from build123d import *

# Parameters (mm, degrees)
SKETCH1_W           = 400
SKETCH1_H           = 20
BOSS_EXTRUDE1_DEPTH = 7.5
SKETCH2_R           = 2.5
BOSS_EXTRUDE2_DEPTH = 75
SKETCH3_R           = 2.5
BOSS_EXTRUDE3_DEPTH = 75
SKETCH5_R           = 10
BOSS_EXTRUDE4_DEPTH = 5
BOSS_EXTRUDE5_START = 20
SKETCH6_R           = 10
BOSS_EXTRUDE5_DEPTH = 20
SKETCH7_R           = 8
CUT_EXTRUDE1_DEPTH  = 15


with BuildPart() as part:
    # Sketch1 → Boss-Extrude1 (new body)
    with BuildSketch(Plane(origin=(0, 0, 0), x_dir=(1, 0, 0), z_dir=(0, 1, 0))):
        Rectangle(SKETCH1_W, SKETCH1_H)
        Polygon((200, 10), (0, 20), (-200, 10), align=None)
        Polygon((0, -20), (-200, -10), (200, -10), align=None)
    extrude(amount=BOSS_EXTRUDE1_DEPTH)

    # Sketch2 → Boss-Extrude2 (add)
    with BuildSketch(Plane(origin=(200, 0, 0), x_dir=(0, 0, -1), z_dir=(1, 0, 0))):
        with Locations((0, 3.296264787)):
            Circle(SKETCH2_R)
    extrude(amount=BOSS_EXTRUDE2_DEPTH)

    # Sketch3 → Boss-Extrude3 (add)
    with BuildSketch(Plane.ZY.offset(200)):
        with Locations((0, 3.469116297)):
            Circle(SKETCH3_R)
    extrude(amount=BOSS_EXTRUDE3_DEPTH)

    # Sketch5 → Boss-Extrude4 (add)
    with BuildSketch(Plane(origin=(0, 7.5, 0), x_dir=(1, 0, 0), z_dir=(0, 1, 0))):
        with Locations(Location((0, 0, 0), (0, 0, 270))):
            Circle(SKETCH5_R)
    extrude(amount=BOSS_EXTRUDE4_DEPTH)

    # Sketch6 → Boss-Extrude5 (add)
    with BuildSketch(Plane.XZ.offset(BOSS_EXTRUDE5_START)):
        with Locations(Location((0, 0, 0), (0, 0, 90))):
            Circle(SKETCH6_R)
    extrude(amount=-BOSS_EXTRUDE5_DEPTH)

    # Sketch7 → Cut-Extrude1 (cut)
    with BuildSketch(Plane(origin=(0, -20, 0), x_dir=(-1, 0, 0), z_dir=(0, -1, 0))):
        with Locations(Location((0, 0, 0), (0, 0, 90))):
            Circle(SKETCH7_R)
    extrude(amount=-CUT_EXTRUDE1_DEPTH, mode=Mode.SUBTRACT)


solid = part.part
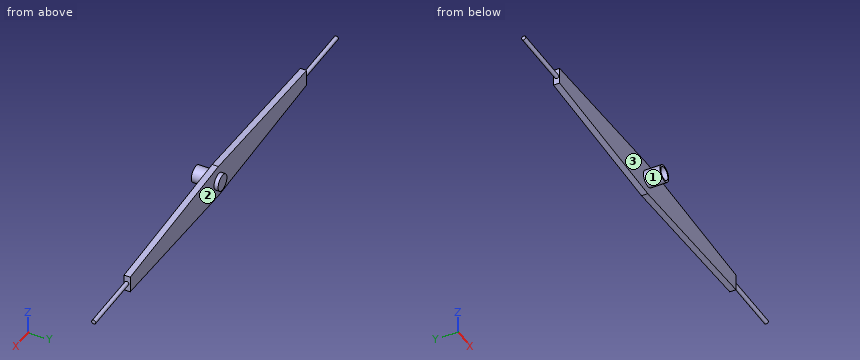
Design review of the part built by this model. Coordinates are the model's own, in mm. Face numbers are marked on the shaded views. Give positions to 0.01 mm unless a question says otherwise; leave off trailing zeros. Write each loop counter-clockwise with the first axis right and the second up, starting at its lowest first coordinate (ties: lowest second). Pieces come first, ordered by that corner, then holes. Notation, with made-up numbers: M 40,62 L 91,62 A6 ccw 91,72 Z; hole C 19.5,22.25 d9. An arc over 180 degrees is marked long. Return JSON: item names as keys, results as strings. Group by question number.
Item 1: Take a section at A-A (x = -34). Give the boundary of the cut face in (y, z).
Item 2: Take a section at B-B (z = 14.5). Give the boundary of the cut face in (x, y).
Item 3: Wall thickness on line 1 along X through (y, z) = (-11.5, 0); line 2 along X through (y, z) = (2, 8); line 3 along Y through (x, z) = (10, 11): over which ranges is each line inside the solid? List them lowest first.
Item 4: The part is to be moulded in two halves that separate along Y. For the marked faces 1, 2 and 3, say which applies: pulls with the +Y half, pulls with the -Y half, needs draft (parallel to the pull), parting line crosses it, or undercut.
Item 5: Clearance check with flat-ended pins moving along their axes: pin 1 Ø6 at (y, z) = (5.5, -3) entering from +X; pin 2 Ø5 at (x, z) = (-0.5, 2) entering from -Y; pin 3 Ø4 at (x, z) = (-152, -11.5) entering from -Y; pin 4 Ø3 at (y, z) = (-11, -0.5) entering from +X. State where each tip first meets the part, or that it passes through.
Item 6: Take a section at C-C (y = -10). Give the boundary of the cut face in (x, z).
Return value:
{
 "1": {"outline": "M 0,-18.3 L 7.5,-18.3 L 7.5,18.3 L 0,18.3 Z"},
 "2": {"outline": "M -110,0 L 110,0 L 110,7.5 L -110,7.5 Z"},
 "3": {"line 1": "x = -10 to -8, 8 to 10", "line 2": "x = -200 to 200", "line 3": "y = 0 to 7.5"},
 "4": {"face 1": "needs draft", "face 2": "pulls with the +Y half", "face 3": "pulls with the -Y half"},
 "5": {"pin 1": "stops at x = 275", "pin 2": "stops at y = -5", "pin 3": "stops at y = 0", "pin 4": "stops at x = 10"},
 "6": {"outline": "C 0,0 d20; hole C 0,0 d16"}
}
